Model file for the job. Use its own axes, mm. A direction names the side the tool comes from. Give positions to 0.01 mm unless a question says otherwise; leave off trailing zeros. Order: outer loops, then holes, each group sorted by start corner. A loop starts at its lowest first (then second) coordinate and runs counter-clockwise, first axis right, second up. Notation, with made-up numbers: M 50,-1.5 L 98,-1.5 A30 ccw 98,28.5 Z; hole C 33.25,-13.5 d5. An arc over 180 degrees is marked long. Return JSON: item names as keys, results as strings. Group by question number.
1. Slice it at D-D on z = -52. List the corners of the cut face in (x, y), then the cut area to 3 significant figures.
2. Pin check, flat tips, straight feed: pin 1 (6.5 mm diameter, centred on y = 313.44, z = -50.6, fed in from +X); pin 2 (11 mm diameter, centred on y = 317.5, z = 0, fed in from -X); pin 3 (1 mm diameter, centred on x = -4.5, y = 319.5, fed in from +Z); pin 4 (8 mm diameter, centred on x = -9.5, y = 308, fed in from +Z). Stop position of each tip, or through.
3. Slice it at B-B on y = 319. List the corners of the cut face in (x, z), then the cut area to 3 significant figures.
4. Wall check: probe 1 along Z at (x, y) = (2.05, 317.5); probe 2 along Z at (x, y) = (1.5, 316.5); probe 3 along X at (y, z) = (316.5, -53). Give the ranges that are in metal, low to high. Write a range as [from, to].
5. Slice it at C-C on x = 1. List the corners of the cut face in (y, z) (1 decimal), then the cut area to 3 significant figures.
6. Slice it at A-A on z = 0. List the corners of the cut face in (x, y), then the cut area to 3 significant figures.
7. 3-axis set-ups, long thin cutter, end or side, ignore diameter. For faces 1 (the face through (-12.7, 317, -25)), 2 (the face through (1.252, 303.783, -24.875)), 3 (the face through (1.252, 329.187, -25.842)), 4 (the face through (-1.967, 313.075, -24.623)), 5 (the face through (-6.261, 310.285, -26.756)): which of +Z, -Z, +X, -X, +Y, -Y reach the whole face in a straight line?
8. Two-plate mould, pull along Z, no slides. Class faces 6 (the face through (1.252, 311.343, -63.127)), 7 (the face through (1.25, 317.07, 12.69)), 8 (the face through (1.252, 320.963, 0.455)), 9 (the face through (2.54, 311, -27)): released by +Z, released by -Z, zero draft, split by the parting line, or undercut.
from build123d import *

# Parameters (mm, degrees)
SKETCH1_R           = 3.4925
BOSS_EXTRUDE1_DEPTH = 2.54
SKETCH2_R           = 6.35
BOSS_EXTRUDE2_DEPTH = 12.7
SKETCH4_R           = 3.4925
CUT_EXTRUDE1_DEPTH  = 6.35


with BuildPart() as part:
    # Sketch1 → Boss-Extrude1 (new body)
    with BuildSketch(Plane(origin=(0, 0, 0), x_dir=(0, 0, -1), z_dir=(1, 0, 0))):
        with BuildLine():
            Line((-12.189561356, 304.55616), (-13.205358136, 329.93584))
            ThreePointArc((-13.205358136, 329.93584), (26.39485874, 329.14336), (65.615293749, 323.615007727))
            Line((65.615293749, 323.615007727), (60.567963461, 298.721545594))
            ThreePointArc((60.567963461, 298.721545594), (24.364484991, 303.82464), (-12.189561356, 304.55616))
        make_face()
        with Locations((0, 317.5)):
            Circle(SKETCH1_R, mode=Mode.SUBTRACT)
        with Locations((25.379671865, 316.484)):
            Circle(SKETCH1_R, mode=Mode.SUBTRACT)
        with Locations((50.596913831, 313.4425024)):
            Circle(SKETCH1_R, mode=Mode.SUBTRACT)
    extrude(amount=BOSS_EXTRUDE1_DEPTH)

    # Sketch2 → Boss-Extrude2 (add)
    with BuildSketch(Plane.ZY):
        with Locations((-25.379671865, 316.484)):
            Circle(SKETCH2_R)
    extrude(amount=BOSS_EXTRUDE2_DEPTH)

    # Sketch4 → Cut-Extrude1 (cut)
    with BuildSketch(Plane(origin=(0, 0, 0), x_dir=(0, 0, -1), z_dir=(1, 0, 0))):
        with Locations((25.379671865, 316.484)):
            Circle(SKETCH4_R)
    extrude(amount=-CUT_EXTRUDE1_DEPTH, mode=Mode.SUBTRACT)


solid = part.part
Result:
{
 "1": {"outline": "M 0,300.33 L 2.54,300.33 L 2.54,310.24 L 0,310.24 Z; M 0,316.64 L 2.54,316.64 L 2.54,326.08 L 0,326.08 Z", "area": "49.2 mm2"},
 "2": {"pin 1": "passes through", "pin 2": "stops at x = 0", "pin 3": "stops at z = -19.55", "pin 4": "stops at z = -20.88"},
 "3": {"outline": "M -12.7,-31.21 L 0,-31.21 L 0,-64.68 L 2.54,-64.68 L 2.54,-27.8 L -6.35,-27.8 L -6.35,-22.96 L 2.54,-22.96 L 2.54,-3.15 L 0,-3.15 L 0,-19.55 L -12.7,-19.55 Z; M 0,3.15 L 2.54,3.15 L 2.54,12.77 L 0,12.77 Z", "area": "286 mm2"},
 "4": {"probe 1": "z = [-64.38, -28.72], [-22.04, -3.49], [3.49, 12.71]", "probe 2": "z = [-64.17, -52.28], [-48.91, -28.87], [-21.89, -3.35], [3.35, 12.67]", "probe 3": "x = [0, 2.54]"},
 "5": {"outline": "M 298.7,-60.6 L 323.6,-65.6 A330.2 ccw 329.9,13.2 L 304.6,12.2 A304.8 cw Z; hole C 313.4,-50.6 d7; hole C 316.5,-25.4 d7; hole C 317.5,0 d7", "area": "1,820 mm2"},
 "6": {"outline": "M 0,304.8 L 2.54,304.8 L 2.54,314.01 L 0,314.01 Z; M 0,320.99 L 2.54,320.99 L 2.54,330.2 L 0,330.2 Z", "area": "46.8 mm2"},
 "7": {"face 1": "+Z, -Z, -X, +Y, -Y", "face 2": "+X, -X, -Y", "face 3": "+X, -X, +Y", "face 4": "+X", "face 5": "-X"},
 "8": {"face 6": "released by -Z", "face 7": "released by +Z", "face 8": "undercut", "face 9": "zero draft"}
}
